from build123d import *

# Parameters (mm, degrees)
F0_W     = 203.2
F0_H     = 127
F1_DEPTH = 127
F3_DEPTH = 76.2
F4_SIZE2 = 101.6
F4_SIZE  = 76.2
F5_R     = 5.08
F6_R     = 15.24
F7_DEPTH = 50.8
F8_R     = 16.51
F9_DEPTH = 127


with BuildPart() as f1:
    # F0 (on Front) → F1 (new body)
    with BuildSketch(Plane.XZ):
        with Locations((0, 2.9180156587)):
            Rectangle(F0_W, F0_H)
    extrude(amount=F1_DEPTH)

    # F2 (on face) → F3 (cut)
    with BuildSketch(Plane.XZ.offset(127)):
        Polygon((-36.9453281164, 0), (-36.9453281164, -60.5819843413), (101.6, -60.5819843413), (101.6, 66.4180156587), (0, 66.4180156587), (0, 0), align=None)
    extrude(amount=-F3_DEPTH, mode=Mode.SUBTRACT)

    # F4
    f4_edges = [f1.edges().sort_by_distance(p)[0] for p in [
        (101.6, -25.4, 66.418016),
    ]]
    f4_side = f1.faces().sort_by_distance((-21.771429, -52.614286, 66.418016))[0]
    chamfer(f4_edges, length=F4_SIZE, length2=F4_SIZE2, reference=f4_side)

    # F5
    f5_edges = [f1.edges().sort_by_distance(p)[0] for p in [
        (-38.1, 0, 66.418016),
        (25.4, -25.4, 66.418016),
        (-101.6, -63.5, 66.418016),
        (12.7, -50.8, 66.418016),
        (-50.8, -127, 66.418016),
        (0, -88.9, 66.418016),
        (0, -88.9, 0),
        (0, -127, 33.209008),
        (0, -50.8, 33.209008),
        (-69.272664, -127, -60.581984),
        (-101.6, -127, 2.918016),
        (-18.472664, -127, 0),
        (-36.945328, -127, -30.290992),
        (-36.945328, -88.9, 0),
        (-36.945328, -88.9, -60.581984),
        (-36.945328, -50.8, -30.290992),
        (-101.6, -63.5, -60.581984),
        (-101.6, 0, 2.918016),
        (32.327336, -50.8, -60.581984),
        (-18.472664, -50.8, 0),
    ]]
    fillet(f5_edges, radius=F5_R)

    # F6 (on face) → F7 (cut, through all)
    with BuildSketch(Plane.XZ.offset(50.8)):
        with Locations((18.9346718836, -14.8619843413)):
            Circle(F6_R)
    extrude(amount=-F7_DEPTH, mode=Mode.SUBTRACT)

    # F8 (on face) → F9 (cut, through all)
    with BuildSketch(Plane.XY.offset(66.4180156587)):
        with Locations((-75.8790969849, -78.356936574)):
            Circle(F8_R)
    extrude(amount=-F9_DEPTH, mode=Mode.SUBTRACT)


solid = f1.part
Input: part model. Units: mm. Frame: model coordinates. A direction names the side the tool comes from. Give positions to 0.01 mm unless a question says otherwise; leave off trailing zeros. Order: outer loops, then holes, each group sorted by start corner. A loop starts at its lowest first (then second) coordinate and runs counter-clockwise, first axis right, second up.
Q1. Section C-C on x = -70. Output: boundary loops of the cut face in (y, z).
Checked values:
outline: (-127, -55.5) arc R5.08 ccw to (-121.92, -60.58) - (-93.78, -60.58) - (-93.78, 66.42) - (-121.92, 66.42) arc R5.08 ccw to (-127, 61.34) - close; (-62.93, -60.58) - (0, -60.58) - (0, 61.34) arc R5.08 ccw to (-5.08, 66.42) - (-62.93, 66.42) - close
Q2. Section A-A on z = -19.5. Output: boundary loops of the cut face in (x, y), and give its area (3 significant figures).
Checked values:
outline: (-101.6, -121.92) arc R5.08 ccw to (-96.52, -127) - (-42.03, -127) arc R5.08 ccw to (-36.95, -121.92) - (-36.95, -55.88) arc R5.08 cw to (-31.87, -50.8) - (4.42, -50.8) - (4.42, 0) - (-96.52, 0) arc R5.08 ccw to (-101.6, -5.08) - close; (33.45, -50.8) - (89.84, -50.8) - (89.84, 0) - (33.45, 0) - close; hole circle Ø33.02 at (-75.88, -78.36)
area: 12,300 mm2
Q3. Draft query along Y for faces 1 (the cylindrical face through (-78.028, -61.987, 3.807)), 2 (the cylindrical face through (-32.77, -1.53, 64.97)), 3 (the flat face through (64.78, -25.04, 13.91)), 4 (the cylindrical face through (-35.42, -52.25, -30.64)). Return one class per face: +Y half, -Y half, draft (parallel to the pull), parting line (faces both ways), or undercut.
Checked values:
face 1: undercut
face 2: +Y half
face 3: draft
face 4: -Y half
Q4. Set-up query: faces 5 (the cylindrical face through (-1.449, -88.438, 1.528)), 6 (the flat face through (0, -89, 34)), 7 (the cylindrical face through (14.29, -49.27, 64.97)), 8 (the flat face through (-21, -33, -60.582)). Return all of +Z, -Z, +X, -X, +Y, -Y with unobstructed straight access to the full face (end or side cutting, diameter ignored); none if empty.
Checked values:
face 5: -Z, +X, -Y
face 6: +Z, -Z, +X, -Y
face 7: +Z, +X, -Y
face 8: -Z, +X, -X, +Y, -Y
Q5. Contact query for flat-ended pins moving along their axis: pin 1 Ø1 at (y, z) = (-35.5, 3) entering from +X; pin 2 Ø8 at (x, y) = (-19.5, -73.5) entering from -Z; pin 3 Ø3 at (x, y) = (61, -27) entering from +Z. Output: stop coordinate, or through.
Checked values:
pin 1: stops at x = 73.34
pin 2: stops at z = 0
pin 3: stops at z = 20.95
Q6. Section B-B on y = -117. Output: boundary loops of the cut face in (x, z).
Checked values:
outline: (-101.6, -55.5) arc R5.08 ccw to (-96.52, -60.58) - (-42.03, -60.58) arc R5.08 ccw to (-36.95, -55.5) - (-36.95, -5.08) arc R5.08 cw to (-31.87, 0) - (-5.08, 0) arc R5.08 ccw to (0, 5.08) - (0, 61.34) arc R5.08 ccw to (-5.08, 66.42) - (-96.52, 66.42) arc R5.08 ccw to (-101.6, 61.34) - close
Q7. Section D-D on z = 7.5. Output: boundary loops of the cut face in (x, y).
Checked values:
outline: (-101.6, -121.92) arc R5.08 ccw to (-96.52, -127) - (-5.08, -127) arc R5.08 ccw to (0, -121.92) - (0, -55.88) arc R5.08 cw to (5.08, -50.8) - (69.59, -50.8) - (69.59, 0) - (-96.52, 0) arc R5.08 ccw to (-101.6, -5.08) - close; hole circle Ø33.02 at (-75.88, -78.36)
Q8. Ray query, probe 1 along X at (y, z) = (-109, 32.5); probe 2 along X at (y, z) = (-104.5, -38); probe 3 along Y at (x, z) = (8, 51). Return the intervals inside material, ascending.
Checked values:
probe 1: x = -101.6 to 0
probe 2: x = -101.6 to -36.95
probe 3: y = -50.8 to 0
